```python
from build123d import *

# Parameters (mm, degrees)
BOSS_EXTRU_1_DEPTH      = 36
ESQUISSE2_W             = 20
ESQUISSE2_H             = 10
ENL_V_MAT_EXTRU_1_DEPTH = 33
ESQUISSE3_W             = 20
ESQUISSE3_H             = 10
ENL_V_MAT_EXTRU_2_DEPTH = 33
ESQUISSE5_W             = 6
ESQUISSE5_H             = 60
BOSS_EXTRU_3_DEPTH      = 20
ESQUISSE6_W             = 3
ESQUISSE6_H             = 60
ENL_V_MAT_EXTRU_3_DEPTH = 50


with BuildPart() as part:
    # Esquisse1 → Boss.-Extru.1 (new body)
    with BuildSketch(Plane.XY):
        Polygon((-21.058577834, 39.100001216), (-44.058577834, 39.100001216), (-44.058577834, -20.899998784), (-21.058577834, -20.899998784), (-21.058577834, -10.899998784), (-41.058577834, -10.899998784), (-41.058577834, 29.100001216), (-21.058577834, 29.100001216), align=None)
    extrude(amount=BOSS_EXTRU_1_DEPTH)

    # Esquisse2 → Enlèv. mat.-Extru.1 (cut)
    with BuildSketch(Plane.XY.offset(36)):
        with Locations((-31.058577834, 34.100001216)):
            Rectangle(ESQUISSE2_W, ESQUISSE2_H)
    extrude(amount=-ENL_V_MAT_EXTRU_1_DEPTH, mode=Mode.SUBTRACT)

    # Esquisse3 → Enlèv. mat.-Extru.2 (cut)
    with BuildSketch(Plane.XY.offset(36)):
        with Locations((-31.058577834, -15.899998784)):
            Rectangle(ESQUISSE3_W, ESQUISSE3_H)
    extrude(amount=-ENL_V_MAT_EXTRU_2_DEPTH, mode=Mode.SUBTRACT)

    # Esquisse5 → Boss.-Extru.3 (add)
    with BuildSketch(Plane(origin=(-41.058577834, 0, 0), x_dir=(0, 0, -1), z_dir=(1, 0, 0))):
        with Locations((-33, 9.100001216)):
            Rectangle(ESQUISSE5_W, ESQUISSE5_H)
    extrude(amount=BOSS_EXTRU_3_DEPTH)

    # Esquisse6 → Enlèv. mat.-Extru.3 (cut)
    with BuildSketch(Plane(origin=(-21.058577834, 0, 0), x_dir=(0, 0, -1), z_dir=(1, 0, 0))):
        with Locations((-34.5, 9.100001216)):
            Rectangle(ESQUISSE6_W, ESQUISSE6_H)
    extrude(amount=-ENL_V_MAT_EXTRU_3_DEPTH, mode=Mode.SUBTRACT)


solid = part.part
```
CAD build for the part. Positions are in the model's coordinates, mm. A direction names the side the tool comes from. Round coordinates to 2 decimals unless told otherwise and drop trailing zeros. Order: outer loops, then holes, each group sorted by start corner. A loop starts at its lowest first (then second) coordinate and runs counter-clockwise, first axis right, second up.
Q1. Slice it at A-A (x = -30.5). Write the cut outline in (y, z), and give its area (3 significant figures).
Q2. Drop flat-ended pins along their axis: pin 1 (10 mm diameter, centred on x = -33, y = 9, fed in from -Z); pin 2 (1.5 mm diameter, centred on y = 23.5, z = 20, fed in from +X). Give the stop position or say it passes through.
Q3. Slice it at D-D (y = 1.5). Write the cut outline in (x, z), and give its area (3 significant figures).
Q4. Two-plate mould, pull along Y, no slides. Class faces 4 (the flat face through (-32, 9, 33)), 5 (the flat face through (-42, -20.9, 19)), 6 (the flat face through (-31, -10.9, 1)): pulls with the +Y half, pulls with the -Y half, needs draft (parallel to the pull), parting line crosses it, or undercut.
Q5. Slice it at C-C (z = 7). Write the cut outline in (x, y), and give its area (3 significant figures).
Q6. Slice it at B-B (y = 32.5). Write the cut outline in (x, z).
Q7. Which spindle directions (+Z, -Z, +X, -X, +Y, -Y) get a long thin tool onto all of the face, cutting with end or side? Do faces 1 (the flat face through (-42, 39.1, 19)), 2 (the flat face through (-31, 9, 30)), 3 (the flat face through (-31, 29.1, 1)). Say none if no direction does.
Q8. Wall check: L1, parallel to Y at x = -40, z = 2; L2, parallel to Z at x = -40, y = 33.5; L3, parallel to X at y = 8.5, z = 9.5. Give the ranges that are in metal, low to high.
Results below:
1. outline: (-20.9, 0) - (-10.9, 0) - (-10.9, 3) - (-20.9, 3) - close; (-20.9, 30) - (39.1, 30) - (39.1, 33) - (-20.9, 33) - close; (29.1, 0) - (39.1, 0) - (39.1, 3) - (29.1, 3) - close
1. area: 240 mm2
2. pin 1: stops at z = 30
2. pin 2: stops at x = -41.06
3. outline: (-44.06, 0) - (-41.06, 0) - (-41.06, 30) - (-21.06, 30) - (-21.06, 33) - (-44.06, 33) - close
3. area: 159 mm2
4. face 4: needs draft
4. face 5: pulls with the -Y half
4. face 6: undercut
5. outline: (-44.06, -20.9) - (-41.06, -20.9) - (-41.06, 39.1) - (-44.06, 39.1) - close
5. area: 180 mm2
6. outline: (-44.06, 0) - (-21.06, 0) - (-21.06, 3) - (-41.06, 3) - (-41.06, 30) - (-21.06, 30) - (-21.06, 33) - (-44.06, 33) - close
7. face 1: +Z, -Z, +X, -X, +Y
7. face 2: +X, +Y, -Y
7. face 3: -Z, +X
8. L1: y = -20.9 to -10.9, 29.1 to 39.1
8. L2: z = 0 to 3, 30 to 33
8. L3: x = -44.06 to -41.06
